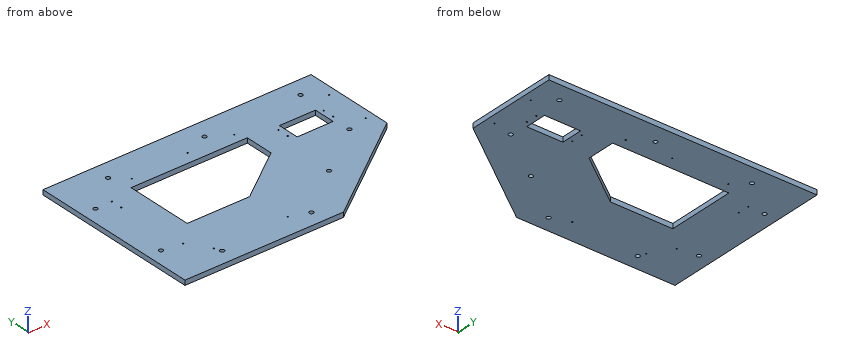
Autodesk Inventor part; units mm, degrees
ref_plane "YZ Plane" through (0, 0, 0) normal (1, 0, 0) x (0, 1, 0)
ref_plane "XZ Plane" through (0, 0, 0) normal (0, 1, 0) x (-1, 0, 0)
ref_plane "XY Plane" through (0, 0, 0) normal (0, 0, 1) x (1, 0, 0)
sketch "Sketch1" plane through (0, 0, 0) normal (0, 0, 1) x (1, 0, 0)
  line L0 (1080.9387, 856.8456) -> (-31.0901, 856.8456)
  line L1 (-31.0901, 856.8456) -> (-31.0901, 139.4979)
  line L2 (-31.0901, 139.4979) -> (626.2703, 139.4979)
  line L3 (626.2703, 139.4979) -> (1080.9387, 473.3358)
  line L4 (1080.9387, 473.3358) -> (1080.9387, 856.8456)
  line L5 (963.1788, 520.0847) -> (751.3683, 364.564) construction
  line L6 (195.0188, 687.1378) -> (677.0148, 687.1378)
  line L7 (677.0148, 687.1378) -> (677.0148, 567.5728)
  line L8 (677.0148, 567.5728) -> (453.8217, 403.6944)
  line L9 (453.8217, 403.6944) -> (195.0188, 403.6944)
  line L10 (195.0188, 403.6944) -> (195.0188, 687.1378)
  line L11 (804.0525, 679.6649) -> (953.5087, 679.6649)
  line L12 (953.5087, 679.6649) -> (953.5087, 589.9913)
  line L13 (953.5087, 589.9913) -> (804.0525, 589.9913)
  line L14 (804.0525, 589.9913) -> (804.0525, 679.6649)
  point P0 (175.6092, 779.9153)
  point P1 (575.6092, 779.9153)
  point P2 (975.6092, 781.6554)
  point P3 (545.6092, 203.1178)
  point P4 (175.6092, 203.1178)
  point P5 (25, 660.086)
  point P6 (25, 328.8534)
  dimension "d1" = 400
  dimension "d2" = 400
  dimension "d3" = 370
extrude "Extrusion1" add sketch "Sketch1" along normal blind 20
sketch "Sketch2" plane through (0, 0, 20) normal (0, 0, 1) x (1, 0, 0)
  point P0 (784.2966, 660.4305)
  point P1 (784.2966, 613.0548)
  point P2 (971.9413, 613.0548)
  point P3 (971.9413, 660.4305)
  point P4 (93.4007, 660.4305)
  point P5 (93.4007, 613.0548)
  point P6 (470.1501, 736.9158)
  point P7 (1046.3575, 723.9381)
  point P8 (1046.3575, 539.6556)
  point P9 (470.1501, 230.7876)
  point P10 (163.8777, 230.7876)
  point P11 (106.776, 316.4401)
  point P12 (656.459, 728.2437)
  point P13 (231.1299, 728.2437)
hole "Hole1" at (784.2966, 660.4305, 20) at (784.2966, 613.0548, 20) at (971.9413, 613.0548, 20) at (971.9413, 660.4305, 20) at (93.4007, 660.4305, 20) at (93.4007, 613.0548, 20) at (470.1501, 736.9158, 20) at (1046.3575, 723.9381, 20) at (1046.3575, 539.6556, 20) at (470.1501, 230.7876, 20) at (163.8777, 230.7876, 20) at (106.776, 316.4401, 20) at (231.1299, 728.2437, 20) at (656.459, 728.2437, 20) direction (0, 0, -1) diameter 5 end through all
sketch "Sketch3" plane through (0, 0, 20) normal (0, 0, 1) x (1, 0, 0)
  line L0 (-31.0901, 139.4979) -> (626.2703, 139.4979)
  line L1 (626.2703, 139.4979) -> (1080.9387, 473.3358)
  line L2 (1080.9387, 473.3358) -> (1080.9387, 856.8456)
  line L3 (963.1788, 520.0847) -> (751.3683, 364.564) construction
  point P0 (175.6092, 779.9153)
  point P1 (575.6092, 779.9153)
  point P2 (975.6092, 781.6554)
  point P3 (545.6092, 203.1178)
  point P4 (175.6092, 203.1178)
  point P5 (25, 660.086)
  point P6 (25, 328.8534)
  dimension "d18" = 400
  dimension "d19" = 400
  dimension "d20" = 370
hole "Hole2" at (25, 328.8534, 20) at (25, 660.086, 20) at (175.6092, 779.9153, 20) at (575.6092, 779.9153, 20) at (975.6092, 781.6554, 20) at (963.1788, 520.0847, 20) at (751.3683, 364.564, 20) at (545.6092, 203.1178, 20) at (175.6092, 203.1178, 20) direction (0, 0, -1) diameter 17.294 end through all
ref_plane "Work Plane1" through (231.1299, 728.2437, 20) normal (1, 0, 0) x (0, 0, -1)
ref_plane "Work Plane2" through (470.1501, 736.9158, -1303.4787) normal (1, 0, 0) x (0, 0, 1)
ref_plane "Work Plane3" through (656.459, 728.2437, 20) normal (1, 0, 0) x (0, 0, -1)
properties part number "plate"
Part model, mm, in its own coordinate system. Give positions to 0.01 mm unless a question says otherwise; leave off trailing zeros. Loops run counter-clockwise (first coordinate to the right, second up) from the corner with the lowest first, then second, coordinate; pieces in that order, holes last. Notation, with made-up numbers: M 80.25,-36 L 127.25,-36 A28 ccw 127.25,-4 Z; hole C -14.75,88 d6. An arc over 180 degrees is marked long. Put each result on its own line as item: value. Start each with the question number.
1) Flat gauge pin, fed straight in: pin 1 (10 mm diameter, centred on x = 851.5, z = 7, fed in from -Y). Where does the tip first touch, or does it go through?
2) Saw through at D-D (y = 263). List the corners of the cut face in (x, z), then the cut area to 3 significant figures.
3) Saw through at A-A (x = 403). List the corners of the cut face in (y, z), then the cut area to 3 significant figures.
4) Saw through at B-B (z = 9.5). State how many separate pieces and enclosed holes the cut face has, then the cut area to 3 significant figures.
5) Probe probe 1 along Y at (x, z) = (94, 8); probe 2 along Y at (x, z) = (231, 14.5); probe 3 along Y at (x, z) = (209, 6.75). List the from-to ranges inside material, lowest first.
6) Saw through at C-C (x = 525). List the corners of the cut face in (y, z), then the cut area to 3 significant figures.
Numbers:
1. pin 1: y = 301.2
2. outline: M -31.09,0 L 794.47,0 L 794.47,20 L -31.09,20 Z
2. area: 16,500 mm^2
3. outline: M 139.5,0 L 403.69,0 L 403.69,20 L 139.5,20 Z; M 687.14,0 L 856.85,0 L 856.85,20 L 687.14,20 Z
3. area: 8,680 mm^2
4. separate pieces: 1
4. enclosed holes: 25
4. area: 588,000 mm^2
5. probe 1: 139.5 to 610.63, 615.48 to 658, 662.86 to 856.85
5. probe 2: 139.5 to 403.69, 687.14 to 725.75, 730.74 to 856.85
5. probe 3: 139.5 to 403.69, 687.14 to 856.85
6. outline: M 139.5,0 L 455.96,0 L 455.96,20 L 139.5,20 Z; M 687.14,0 L 856.85,0 L 856.85,20 L 687.14,20 Z
6. area: 9,720 mm^2
